CAD build for the part. Positions are in the model's coordinates, mm. A direction names the side the tool comes from. Round coordinates to 2 decimals unless told otherwise and drop trailing zeros. Order: outer loops, then holes, each group sorted by start corner. A loop starts at its lowest first (then second) coordinate and runs counter-clockwise, first axis right, second up. Notation, with made-up numbers: (19, 61.25) - (29, 61.25) arc R18 ccw to (29, 65.25) - close; hole circle Ø9 at (77.25, 44.5). An arc over 180 degrees is marked (long way). Use one line per item in the form item = value. Start each with the question number.
from build123d import *

# Parameters (mm, degrees)
SKETCH004_R        = 6
POCKET_DEPTH       = 639.959465
POLARPATTERN_COUNT = 6


with BuildPart() as part:
    # Sketch002 → Revolution003 (revolve)
    with BuildSketch(Plane.XZ):
        Polygon((90, 28), (110, 28), (110, 38), (90, 38), (90, 58), (80, 58), (80, 44), (74.400894, 44), (74.400894, 39), (86, 39), (86, 24), (90, 24), align=None)
    revolve(axis=Axis((0, 0, 0), (0, 0, 1)))

    # Sketch004 (on Face8 of Revolution003) → Pocket (cut, through all)
    with BuildSketch(Plane(origin=(0, 0, 38), x_dir=(-1, 0, 0), z_dir=(0, 0, 1))):
        with Locations((100, 0)):
            Circle(SKETCH004_R)
    pocket = extrude(amount=-POCKET_DEPTH, mode=Mode.SUBTRACT)

    # PolarPattern: Pocket ×6 about axis
    polarpattern_axis = Axis((0, 0, 38), (0, 0, 1))
    for i in range(1, POLARPATTERN_COUNT):
        add(pocket.rotate(polarpattern_axis, i * 360 / POLARPATTERN_COUNT), mode=Mode.SUBTRACT)


solid = part.part
(1) Wall check: line 1 (Y direction, x = 0, z = 32); line 2 (Y direction, x = 0, z = 41.2); line 3 (X direction, y = 3, z = 31.5). Give the ranges that are in metal, low to high. Write a range as [from, to].
(2) Which spindle directions (+Z, -Z, +X, -X, +Y, -Y) get a long thin tool onto all of the face, cutting with end or side? Do faces 4 (the cylindrical face through (41.53, -79.845, 26.028)), 5 (the cylindrical face through (-51.3, -92.46, 33.07)), 6 (the cylindrical face through (-17.34, -78.1, 50.9)). Say none if no direction does.
(3) Flat gauge pins, fed straight in: P1, Ø15.5, axis at x = 100, y = 0, coming from the -Z side; P2, Ø9.5, axis at x = -50, y = 86.6, coming from the -Z side; P3, Ø2, axis at x = 76, z = 39.5, coming from the +Y side; P4, Ø5, axis at x = -84, z = 47.5, coming from the +Y side. Where does each tip first touch, or does it go through?
(4) Slice it at B-B (y = 0). Give the number of separate pieces and of enclosed holes in the cut face, and give its area (3 significant figures).
(5) Slice it at A-A (x = 0). Give the cut face in (y, z).
(6) Mould opens along Y. For faces 1 (the cylindrical face through (41.53, -79.845, 48.14)), 2 (the cylindrical face through (94, 0, 33)), 3 (the flat face through (-8, 90, 28)) say: pulls with the +Y half, pulls with the -Y half, needs draft (parallel to the pull), parting line crosses it, or undercut.
(7) Slice it at D-D (y = -27). Give the cut face in (x, z).
Results list:
q1.line_1 = [-110, -86], [86, 110]
q1.line_2 = [-90, -74.4], [74.4, 90]
q1.line_3 = [-109.96, -105.2], [-94.8, -85.95], [85.95, 94.8], [105.2, 109.96]
q2.face_4 = -Z
q2.face_5 = +Z, -Z
q2.face_6 = +Z
q3.P1 = 28
q3.P2 = through
q3.P3 = 49.75
q3.P4 = 38.18
q4.separate_pieces = 4
q4.enclosed_holes = 0
q4.area = 716 mm²
q5.outline = (-110, 28) - (-90, 28) - (-90, 24) - (-86, 24) - (-86, 39) - (-74.4, 39) - (-74.4, 44) - (-80, 44) - (-80, 58) - (-90, 58) - (-90, 38) - (-110, 38) - close; (74.4, 39) - (86, 39) - (86, 24) - (90, 24) - (90, 28) - (110, 28) - (110, 38) - (90, 38) - (90, 58) - (80, 58) - (80, 44) - (74.4, 44) - close
q6.face_1 = parting line crosses it
q6.face_2 = undercut
q6.face_3 = needs draft
q7.outline = (-106.63, 28) - (-85.85, 28) - (-85.85, 24) - (-81.65, 24) - (-81.65, 39) - (-69.33, 39) - (-69.33, 44) - (-75.31, 44) - (-75.31, 58) - (-85.85, 58) - (-85.85, 38) - (-106.63, 38) - close; (69.33, 39) - (81.65, 39) - (81.65, 24) - (85.85, 24) - (85.85, 28) - (106.63, 28) - (106.63, 38) - (85.85, 38) - (85.85, 58) - (75.31, 58) - (75.31, 44) - (69.33, 44) - close
